The listing builds one solid part. Answer for the finished solid, in the listing's coordinates (mm). A direction names the side the tool comes from. Coordinates: 2 decimals unless noted, no trailing zeros. Write each loop counter-clockwise with the first axis right and the second up, starting at its lowest first coordinate (ties: lowest second). Pieces come first, ordered by that corner, then holes.
(1) The part is cut by section B-B on x = 0. Determine the outline of the cut face in (y, z), plus the area to 3 significant figures.
(2) For a pull along Z with two mould halves and no side action, classify faces 4 (the flat face through (0, 11.8, 0)), 5 (the flat face through (-2.4, 1.3, -1.9)), 6 (the cylindrical face through (-5.158, 0.641, 3.955)) as +Z half, -Z half, draft (parallel to the pull), parting line (faces both ways), or undercut.
(3) The part is cut by section C-C on z = 0. Determine the outline of the cut face in (x, y).
(4) Given P1, Ø1.5, axis at x = -2, y = 6, coming from the -Z side; P2, Ø4, axis at x = -2.5, y = 8, coming from the -Z side; P3, Ø1, axis at x = -4, y = 1, coming from the -Z side; P4, Ø1, axis at x = -3, z = 0, coming from the -Y side, each flat-ended and moving along its own axis, determine where each tip first touches the part or whether it passes through.
(5) Straight lines are drawn through the part: line 1 (Z direction, x = -2.25, y = 1.25); line 2 (Z direction, x = 3.5, y = 2.5); line 3 (Z direction, x = 0, y = 8). For each, find the intervals that lie inside material, in ascending order.
(6) Which of the six approach directions +Z, -Z, +X, -X, +Y, -Y give full straight-line access (tool end or side, diameter ignored) to faces 1 (the cylindrical face through (-5.794, 6.381, -0.255)), 2 (the flat face through (1.9, 2, 0)), 3 (the flat face through (0.3, 2, 4))?
from build123d import *

# Parameters (mm, degrees)
SKETCH1_R           = 6.5
BOSS_EXTRUDE1_DEPTH = 1.5
SKETCH2_R           = 5.8
BOSS_EXTRUDE2_DEPTH = 10.3
FILLET1_R           = 0.4
SKETCH3_R           = 5
CUT_EXTRUDE1_DEPTH  = 4.8
BOSS_EXTRUDE3_DEPTH = 4.8
SKETCH5_W           = 2
SKETCH5_H           = 0.8
SKETCH5_W_2         = 1
SKETCH5_H_2         = 3.8
BOSS_EXTRUDE4_DEPTH = 7.2
CUT_EXTRUDE2_REACH  = 10.4
BOSS_EXTRUDE5_DEPTH = 3.8
FILLET2_R           = 0.1
FILLET3_R           = 0.2


with BuildPart() as part:
    # Sketch1 → Boss-Extrude1 (new body)
    with BuildSketch(Plane(origin=(0, 0, 0), x_dir=(1, 0, 0), z_dir=(0, 1, 0))):
        Circle(SKETCH1_R)
    extrude(amount=BOSS_EXTRUDE1_DEPTH)

    # Sketch2 → Boss-Extrude2 (add)
    with BuildSketch(Plane(origin=(0, 1.5, 0), x_dir=(1, 0, 0), z_dir=(0, 1, 0))):
        Circle(SKETCH2_R)
    extrude(amount=BOSS_EXTRUDE2_DEPTH)

    # Fillet1
    fillet1_edges = [part.edges().sort_by_distance(p)[0] for p in [
        (-5.8, 11.8, 0),
    ]]
    fillet(fillet1_edges, radius=FILLET1_R)

    # Sketch3 → Cut-Extrude1 (cut)
    with BuildSketch(Plane.XZ):
        Circle(SKETCH3_R)
    extrude(amount=-CUT_EXTRUDE1_DEPTH, mode=Mode.SUBTRACT)

    # Sketch4 → Boss-Extrude3 (add)
    with BuildSketch(Plane.XZ.offset(-4.8)):
        with BuildLine():
            Line((-4.990991885, 0.3), (-2.9, 0.3))
            Line((-2.9, 0.3), (-2.9, -0.3))
            Line((-2.9, -0.3), (-4.990991885, -0.3))
            ThreePointArc((-4.990991885, -0.3), (-5, 0), (-4.990991885, 0.3))
        make_face()
        with BuildLine():
            Line((2.9, 0.3), (2.9, -0.3))
            Line((2.9, -0.3), (4.990991885, -0.3))
            ThreePointArc((4.990991885, -0.3), (5, 0), (4.990991885, 0.3))
            Line((4.990991885, 0.3), (2.9, 0.3))
        make_face()
        with BuildLine():
            Line((-0.3, 4.990991885), (-0.3, 2.7))
            Line((-0.3, 2.7), (0.3, 2.7))
            Line((0.3, 2.7), (0.3, 4.990991885))
            ThreePointArc((0.3, 4.990991885), (0, 5), (-0.3, 4.990991885))
        make_face()
        with BuildLine():
            Line((0.3, -2.7), (-0.3, -2.7))
            Line((-0.3, -2.7), (-0.3, -4.990991885))
            ThreePointArc((-0.3, -4.990991885), (0, -5), (0.3, -4.990991885))
            Line((0.3, -4.990991885), (0.3, -2.7))
        make_face()
    extrude(amount=BOSS_EXTRUDE3_DEPTH)

    # Sketch5 → Boss-Extrude4 (add)
    with BuildSketch(Plane.XZ.offset(-4.8)):
        with Locations((0, 2.3)):
            Rectangle(SKETCH5_W, SKETCH5_H)
        with Locations((-2.4, 0)):
            Rectangle(SKETCH5_W_2, SKETCH5_H_2)
        with Locations((2.4, 0)):
            Rectangle(SKETCH5_W_2, SKETCH5_H_2)
        with Locations((0, -2.3)):
            Rectangle(SKETCH5_W, SKETCH5_H)
    extrude(amount=BOSS_EXTRUDE4_DEPTH)

    # Sketch6 → Cut-Extrude2 (cut, up to next)
    with BuildSketch(Plane.XY.offset(1.9), mode=Mode.PRIVATE) as cut_extrude2_sk1:
        Polygon((-1.9, -2.4), (-1.9, -1.9625), (-2.4, -2.4), align=None)
    cut_extrude2_tool1 = extrude(cut_extrude2_sk1.sketch, amount=-CUT_EXTRUDE2_REACH, mode=Mode.PRIVATE) & part.part
    add(cut_extrude2_tool1.solids().sort_by_distance((-2.066667, -2.254167, 1.9))[0], mode=Mode.SUBTRACT)
    # Sketch6 → Cut-Extrude2 (cut, up to next)
    with BuildSketch(Plane.XY.offset(1.9), mode=Mode.PRIVATE) as cut_extrude2_sk2:
        Polygon((1.9, -1.9625), (1.9, -2.4), (2.4, -2.4), align=None)
    cut_extrude2_tool2 = extrude(cut_extrude2_sk2.sketch, amount=-CUT_EXTRUDE2_REACH, mode=Mode.PRIVATE) & part.part
    add(cut_extrude2_tool2.solids().sort_by_distance((2.066667, -2.254167, 1.9))[0], mode=Mode.SUBTRACT)

    # Sketch6<3> → Boss-Extrude5 (add)
    with BuildSketch(Plane.XY.offset(1.9)):
        Polygon((-1.6, -1.7), (-1.9, -1.4), (-1.9, -1.9625), align=None)
        Polygon((1.6, -1.7), (1.9, -1.9625), (1.9, -1.4), align=None)
    extrude(amount=-BOSS_EXTRUDE5_DEPTH)

    # Fillet2
    fillet2_edges = [part.edges().sort_by_distance(p)[0] for p in [
        (-1.6, -1.7, 0),
        (1.6, -1.7, 0),
    ]]
    fillet(fillet2_edges, radius=FILLET2_R)

    # Fillet3
    fillet3_edges = [part.edges().sort_by_distance(p)[0] for p in [
        (-6.5, 1.5, 0),
    ]]
    fillet(fillet3_edges, radius=FILLET3_R)


solid = part.part
Model answer:
1. outline: (-2.4, -2.7) - (0, -2.7) - (0, -6.5) - (1.3, -6.5) arc R0.2 ccw to (1.5, -6.3) - (1.5, -5.8) - (11.4, -5.8) arc R0.4 ccw to (11.8, -5.4) - (11.8, 5.4) arc R0.4 ccw to (11.4, 5.8) - (1.5, 5.8) - (1.5, 6.3) arc R0.2 ccw to (1.3, 6.5) - (0, 6.5) - (0, 2.7) - (-2.4, 2.7) - (-2.4, 1.9) - (4.8, 1.9) - (4.8, -1.9) - (-2.4, -1.9) - close
1. area: 124 mm2
2. face 4: draft
2. face 5: undercut
2. face 6: parting line
3. outline: (-6.5, 0) - (-2.9, 0) - (-2.9, -2.4) - (-2.4, -2.4) - (-1.68, -1.77) arc R0.1 ccw to (-1.68, -1.62) - (-1.9, -1.4) - (-1.9, 4.8) - (1.9, 4.8) - (1.9, -1.4) - (1.68, -1.62) arc R0.1 ccw to (1.68, -1.77) - (2.4, -2.4) - (2.9, -2.4) - (2.9, 0) - (6.5, 0) - (6.5, 1.3) arc R0.2 ccw to (6.3, 1.5) - (5.8, 1.5) - (5.8, 11.4) arc R0.4 ccw to (5.4, 11.8) - (-5.4, 11.8) arc R0.4 ccw to (-5.8, 11.4) - (-5.8, 1.5) - (-6.3, 1.5) arc R0.2 ccw to (-6.5, 1.3) - close
4. P1: stops at z = -5.66
4. P2: stops at z = -5.78
4. P3: stops at z = -5.48
4. P4: stops at y = -2.4
5. line 1: z = -6.1 to -4.47, -1.9 to 1.9, 4.47 to 6.1
5. line 2: z = -4.62 to -3.57, -0.3 to 0.3, 3.57 to 4.62
5. line 3: z = -5.8 to 5.8
6. face 1: +Y
6. face 2: none
6. face 3: -Y
